Input: part model. Units: mm. Frame: model coordinates. Face numbers are marked on the shaded views. A direction names the side the tool comes from. Round coordinates to 2 decimals unless told otherwise and drop trailing zeros. Loops run counter-clockwise (first coordinate to the right, second up) from the corner with the lowest first, then second, coordinate; pieces in that order, holes last. Notation, with made-up numbers: M -26,24 L 4,24 A32 ccw 4,61 Z; hole C 42,25 d8. An arc over 180 degrees is marked long. Put each result on its own line as item: value. Start each with the question number.
1) Section D-D on z = -3. Output: boundary loops of the cut face in (x, y).
2) Section C-C on z = -7. State how many separate pieces and enclosed holes the cut face has, plus the area to 3 significant figures.
3) Section A-A on x = 45.5. Output: boundary loops of the cut face in (y, z).
4) Reachability of the marked faces 5, 6 and 7 from +Z, -Z, +X, -X, +Y, -Y: full face, straight path, thin tool, end or side. Return the list, or none.
5) Section B-B on y = 17.75. Output: boundary loops of the cut face in (x, z), plus the area to 3 significant figures.
6) Pin query (flat end, axial travel): pin 1 (4 mm diameter, centred on x = 31.686, z = -3, fed in from +Y); pin 2 (8 mm diameter, centred on y = 7.5, z = -8.5, fed in from +X); pin 3 (2 mm diameter, centred on x = 40, y = 15, fed in from -Z); pin 4 (7 mm diameter, centred on y = 22.4, z = -7, fed in from -X). Return the tip coordinate at first contact, or that it passes through.
7) Draft query along X for the marked faces 1, 2, 3 and 4. Return one class per face: +X half, -X half, draft (parallel to the pull), parting line (faces both ways), or undercut.
8) Line query: probe 1 along X at (y, z) = (24, -4); probe 2 along X at (y, z) = (1.5, -3); probe 3 along Y at (x, z) = (12.55, -7). Output: solid intervals per line, ascending.
from build123d import *

# Parameters (mm, degrees)
SKETCH1_W           = 51
SKETCH1_H           = 14
SKETCH1_R           = 2.7
BOSS_EXTRUDE1_DEPTH = 3
SKETCH2_W           = 2.4
SKETCH2_H           = 14
BOSS_EXTRUDE2_DEPTH = 25.4
CUT_EXTRUDE1_REACH  = 5
SKETCH3_R           = 1.25
SKETCH4_R           = 2.65
CUT_EXTRUDE2_DEPTH  = 40.9
CUT_EXTRUDE3_DEPTH  = 40.9
FILLET1_R           = 1
FILLET2_R           = 0.5


with BuildPart() as part:
    # Sketch1 → Boss-Extrude1 (new body)
    with BuildSketch(Plane(origin=(0, 0, 0), x_dir=(1, 0, 0), z_dir=(0, 1, 0))):
        with Locations((25.5, 7)):
            Rectangle(SKETCH1_W, SKETCH1_H)
        with Locations((45.5, 7)):
            Circle(SKETCH1_R, mode=Mode.SUBTRACT)
        with BuildLine():
            Line((4.1, 10), (6.9, 10))
            ThreePointArc((6.9, 10), (9.9, 7), (6.9, 4))
            Line((6.9, 4), (4.1, 4))
            ThreePointArc((4.1, 4), (1.1, 7), (4.1, 10))
        make_face(mode=Mode.SUBTRACT)
    extrude(amount=BOSS_EXTRUDE1_DEPTH)

    # Sketch2 → Boss-Extrude2 (add)
    with BuildSketch(Plane(origin=(0, 3, 0), x_dir=(1, 0, 0), z_dir=(0, 1, 0))):
        with Locations((12.3, 7)):
            Rectangle(SKETCH2_W, SKETCH2_H)
        with Locations((38.7, 7)):
            Rectangle(SKETCH2_W, SKETCH2_H)
    extrude(amount=BOSS_EXTRUDE2_DEPTH)

    # Sketch3 → Cut-Extrude1 (cut, up to next)
    with BuildSketch(Plane(origin=(0, 3, 0), x_dir=(1, 0, 0), z_dir=(0, 1, 0)), mode=Mode.PRIVATE) as cut_extrude1_sk1:
        with Locations((22.314, 3)):
            Circle(SKETCH3_R)
    cut_extrude1_tool1 = extrude(cut_extrude1_sk1.sketch, amount=-CUT_EXTRUDE1_REACH, mode=Mode.PRIVATE) & part.part
    add(cut_extrude1_tool1.solids().sort_by_distance((22.314, 3, -3))[0], mode=Mode.SUBTRACT)
    # Sketch3 → Cut-Extrude1 (cut, up to next)
    with BuildSketch(Plane(origin=(0, 3, 0), x_dir=(1, 0, 0), z_dir=(0, 1, 0)), mode=Mode.PRIVATE) as cut_extrude1_sk2:
        with Locations((31.686, 3)):
            Circle(SKETCH3_R)
    cut_extrude1_tool2 = extrude(cut_extrude1_sk2.sketch, amount=-CUT_EXTRUDE1_REACH, mode=Mode.PRIVATE) & part.part
    add(cut_extrude1_tool2.solids().sort_by_distance((31.686, 3, -3))[0], mode=Mode.SUBTRACT)

    # Sketch4 → Cut-Extrude2 (cut, through all)
    with BuildSketch(Plane.ZY.offset(-11.1)):
        with Locations((-7, 22.4)):
            Circle(SKETCH4_R)
    extrude(amount=-CUT_EXTRUDE2_DEPTH, mode=Mode.SUBTRACT)

    # Sketch5 → Cut-Extrude3 (cut, through all)
    with BuildSketch(Plane.ZY.offset(-11.1)):
        Polygon((-14, 22.4), (-9.798754771, 28.4), (-14, 28.4), align=None)
        Polygon((0, 22.4), (-4.201245229, 28.4), (0, 28.4), align=None)
    extrude(amount=-CUT_EXTRUDE3_DEPTH, mode=Mode.SUBTRACT)

    # Fillet1
    fillet1_edges = [part.edges().sort_by_distance(p)[0] for p in [
        (39.9, 3, -7),
        (11.1, 3, -7),
    ]]
    fillet(fillet1_edges, radius=FILLET1_R)

    # Fillet2
    fillet2_edges = [part.edges().sort_by_distance(p)[0] for p in [
        (37.5, 3, -7),
        (13.5, 3, -7),
    ]]
    fillet(fillet2_edges, radius=FILLET2_R)


solid = part.part
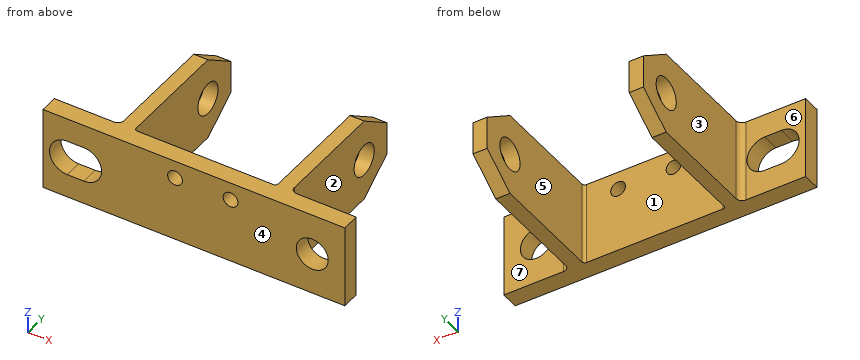
Geometry results:
1. outline: M 0,0 L 21.06,0 L 21.06,3 L 14,3 A0.5 cw 13.5,3.5 L 13.5,26.68 L 11.1,26.68 L 11.1,4 A1 cw 10.1,3 L 0,3 Z; M 23.56,0 L 30.44,0 L 30.44,3 L 23.56,3 Z; M 32.94,0 L 51,0 L 51,3 L 40.9,3 A1 cw 39.9,4 L 39.9,26.68 L 37.5,26.68 L 37.5,3.5 A0.5 cw 37,3 L 32.94,3 Z
2. separate pieces: 5
2. enclosed holes: 0
2. area: 207 mm²
3. outline: M 0,-14 L 3,-14 L 3,-9.7 L 0,-9.7 Z; M 0,-4.3 L 3,-4.3 L 3,0 L 0,0 Z
4. face 5: +Z, -Z, +Y
4. face 6: +Z, -Z, -X, +Y
4. face 7: +Z, -Z, +X, +Y
5. outline: M 11.1,-14 L 13.5,-14 L 13.5,0 L 11.1,0 Z; M 37.5,-14 L 39.9,-14 L 39.9,0 L 37.5,0 Z
5. area: 67.2 mm²
6. pin 1: stops at y = 3
6. pin 2: stops at x = 40.03
6. pin 3: stops at z = -14
6. pin 4: stops at x = 11.1
7. face 1: undercut
7. face 2: +X half
7. face 3: -X half
7. face 4: draft
8. probe 1: x = 11.1 to 13.5, 37.5 to 39.9
8. probe 2: x = 0 to 21.06, 23.56 to 30.44, 32.94 to 51
8. probe 3: y = 0 to 19.75, 25.05 to 28.4
